Input: part model. Units: mm. Frame: model coordinates. Face numbers are marked on the shaded views. A direction names the side the tool comes from. Coordinates: 2 decimals unless noted, no trailing zeros. Write each loop counter-clockwise with the first axis right and the second up, starting at its lowest first coordinate (ties: lowest second). Pieces come first, ordered by that corner, then holes. Notation, with made-up numbers: M -6.5,4.5 L 28.5,4.5 A22 cw 28.5,26.5 Z; hole C -10,-26 d2. An arc over 180 degrees is marked long. Write each question's results on one line, items separated by ' | '. Start each with the question number.
1. Ray query, probe 1 along X at (y, z) = (-39, -13.25); probe 2 along Z at (x, y) = (-79, -30). Return the intervals inside material, ascending.
2. Section query C-C, the plane z = -10.25. Output: boundary loops of the cut face in (x, y), and give its area (3 significant figures).
3. First-contact query: pin 1 (25 mm diameter, centred on x = -36, y = -72, fed in from -Z); pin 2 (6 mm diameter, centred on x = -14.5, z = -1, fed in from +Y); pin 3 (7.5 mm diameter, centred on y = -52, z = -9, fed in from +X). Flat tips, straight axial feed; report the tip coordinate or a pass-through.
4. Section query A-A, the plane y = -28.5. Output: boundary loops of the cut face in (x, z), and give its area (3 significant figures).
5. Section query B-B, the plane x = -71. Output: boundary loops of the cut face in (y, z).
6. Set-up query: the marked faces 1 and 2. Return all of +Z, -Z, +X, -X, +Y, -Y with unobstructed straight access to the full face (end or side cutting, diameter ignored); none if empty.
```python
from build123d import *

# Parameters (mm, degrees)
BOSS_EXTRUDE1_DEPTH = 0.8
BOSS_EXTRUDE2_DEPTH = 0.8
BOSS_EXTRUDE3_DEPTH = 15.4


with BuildPart() as part:
    # Sketch1 → Boss-Extrude1 (new body)
    with BuildSketch(Plane.XY):
        Polygon((2.591679003, 2.54), (2.591679003, -124.46), (-72.414230485, -124.46), (-72.414230485, -121.92), (-72.414230485, 2.54), align=None)
    extrude(amount=BOSS_EXTRUDE1_DEPTH)

    # Sketch2 → Boss-Extrude2 (add)
    with BuildSketch(Plane.XY):
        Polygon((-72.414230485, -124.46), (-80.414230485, -124.46), (-82.954230485, -124.46), (-82.954230485, -112.46), (-82.954230485, 2.54), (-72.414230485, 2.54), (-72.414230485, -9.46), (-72.414230485, -112.46), align=None)
    extrude(amount=BOSS_EXTRUDE2_DEPTH)

    # Sketch3 → Boss-Extrude3 (add)
    with BuildSketch(Plane(origin=(0, 0, 0), x_dir=(-1, 0, 0), z_dir=(0, 0, -1))):
        Polygon((82.954230485, 2.54), (80.414230485, 2.54), (80.414230485, -9.46), (80.414230485, -112.46), (80.414230485, -124.46), (82.954230485, -124.46), (82.954230485, -112.46), (82.954230485, -9.46), align=None)
    extrude(amount=BOSS_EXTRUDE3_DEPTH)


solid = part.part
```
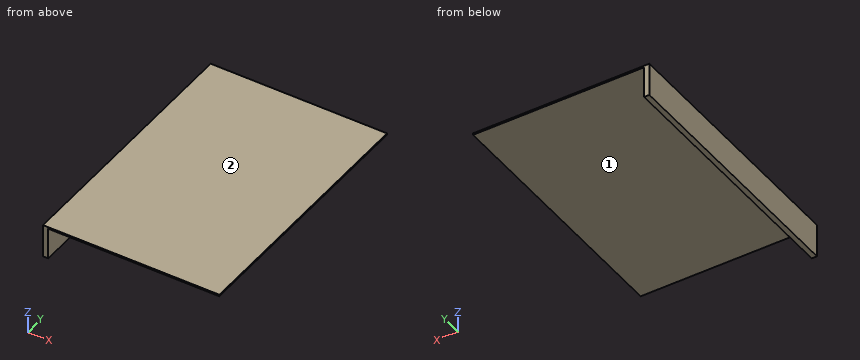
Answer:
1) probe 1: -82.95 to -80.41 | probe 2: 0 to 0.8
2) outline: M -82.95,-124.46 L -80.41,-124.46 L -80.41,2.54 L -82.95,2.54 Z | area: 323 mm^2
3) pin 1: z = 0 | pin 2: y = 2.54 | pin 3: x = -80.41
4) outline: M -82.95,-15.4 L -80.41,-15.4 L -80.41,0 L 2.59,0 L 2.59,0.8 L -82.95,0.8 Z | area: 108 mm^2
5) outline: M -124.46,0 L 2.54,0 L 2.54,0.8 L -124.46,0.8 Z
6) face 1: -Z, +X, +Y, -Y | face 2: +Z, +X, -X, +Y, -Y
